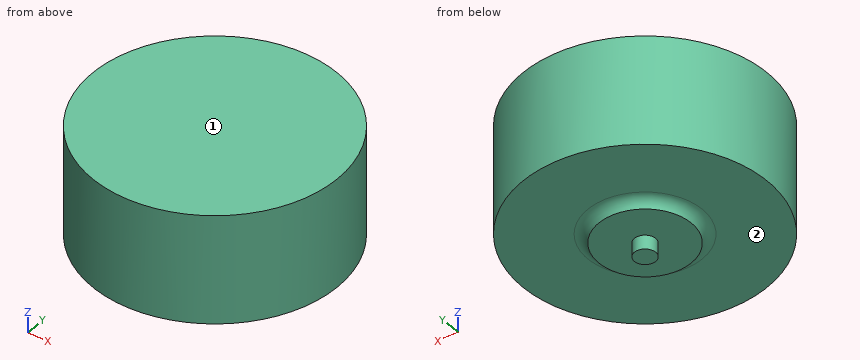
Autodesk Inventor part; units mm, degrees
ref_plane "YZ Plane" through (0, 0, 0) normal (1, 0, 0) x (0, 1, 0)
ref_plane "XZ Plane" through (0, 0, 0) normal (0, 1, 0) x (-1, 0, 0)
ref_plane "XY Plane" through (0, 0, 0) normal (0, 0, 1) x (1, 0, 0)
sketch "Sketch1" plane through (0, 0, 0) normal (0, 0, 1) x (1, 0, 0)
  circle A0 centre (0, 0) radius 34.4
  dimension "d0" = 68.8
extrude "Extrusion1" add sketch "Sketch1" along normal blind 30.5
sketch "Sketch2" plane through (0, 0, 0) normal (0, 0, -1) x (-1, 0, 0)
  circle A0 centre (0, 0) radius 13
  dimension "d3" = 26
extrude "Extrusion2" add sketch "Sketch2" along normal blind 2.5
sketch "Sketch3" plane through (0, 0, -2.5) normal (0, 0, -1) x (-1, 0, 0)
  circle A0 centre (0, 0) radius 3
  dimension "d6" = 6
extrude "Extrusion3" add sketch "Sketch3" along normal blind 3.9
fillet "Fillet1" radius 3.175 1 edges at (13, 0, 0)
properties part number "Motor" material "Copper"
Could you check a few things on this model? Use its own coordinates, in mm. Face numbers are marked on the shaded views. A direction names the side the tool comes from. Round coordinates to 2 decimals unless told otherwise and drop trailing zeros. Write each loop counter-clockwise with the first axis right and the second up, starting at its lowest first coordinate (ties: lowest second). Pieces come first, ordered by that corner, then holes. Notation, with made-up numbers: (29.5, 76) - (68.5, 76) arc R10 cw to (68.5, 94) - close; hole circle Ø4 at (47.5, 23). An arc over 180 degrees is marked (long way). Put each result on its own line as item: value. Start each with the question number.
(1) For the marked faces 1 and 2, which set-ups out of +Z, -Z, +X, -X, +Y, -Y let a thin tool reach every point of the face, with its end or its side?
(2) I want a section at D-D, the plane y = -24. Please give me the cut outline in (x, z).
(3) I need wall thicknesses on probe 1 along Z at (x, y) = (19.5, 11); probe 2 along Z at (x, y) = (-4.5, -9); probe 3 along Y at (x, z) = (-29, 22). Which ranges of each line are inside material? Lowest first, please.
(4) I want a section at C-C, the plane z = 22. Please give me the cut outline in (x, y).
(5) I want a section at A-A, the plane y = 0. Please give me the cut outline in (x, z) (3 decimals), plus the area to 3 significant figures.
(6) Will these pins go through, and if not, where does the flat tip stop? pin 1 (12 mm diameter, centred on y = -14, z = 11.5, fed in from -X); pin 2 (5 mm diameter, centred on y = -22, z = 21.5, fed in from -X); pin 3 (4 mm diameter, centred on x = -23, y = 16, fed in from -Z).
Here are the results:
1. face 1: +Z, +X, -X, +Y, -Y
1. face 2: -Z
2. outline: (-24.64, 0) - (24.64, 0) - (24.64, 30.5) - (-24.64, 30.5) - close
3. probe 1: z = 0 to 30.5
3. probe 2: z = -2.5 to 30.5
3. probe 3: y = -18.5 to 18.5
4. outline: circle Ø68.8 at (0, 0)
5. outline: (-34.4, 0) - (-16.102, 0) arc R3.175 cw to (-13, -2.5) - (-3, -2.5) - (-3, -6.4) - (3, -6.4) - (3, -2.5) - (13, -2.5) arc R3.175 cw to (16.102, 0) - (34.4, 0) - (34.4, 30.5) - (-34.4, 30.5) - close
5. area: 2,190 mm^2
6. pin 1: stops at x = -33.46
6. pin 2: stops at x = -28.34
6. pin 3: stops at z = 0
